Autodesk Inventor part; units mm, degrees
ref_plane "YZ Plane" through (0, 0, 0) normal (1, 0, 0) x (0, 1, 0)
ref_plane "XZ Plane" through (0, 0, 0) normal (0, 1, 0) x (-1, 0, 0)
ref_plane "XY Plane" through (0, 0, 0) normal (0, 0, 1) x (1, 0, 0)
sketch "Sketch1" plane through (0, 0, 0) normal (1, 0, 0) x (0, 1, 0)
  line L0 (32.5, 25) -> (-32.5, 25)
  line L1 (-32.5, 25) -> (-32.5, -25)
  line L2 (-32.5, -25) -> (32.5, -25)
  line L3 (32.5, -25) -> (32.5, 25)
  point P0 (0, 0)
  dimension "d0" = 65
  dimension "d1" = 50
  dimension "d2" = 32.5
  dimension "d3" = 25
extrude "Extrusion1" add sketch "Sketch1" along normal blind 7.5
sketch "Sketch2" plane through (7.5, 0, 0) normal (1, 0, 0) x (0, 0, -1)
  circle A0 centre (-12.5, 20) radius 1.6
  line L0 (25, 32.5) -> (-25, 32.5)
  line L1 (-25, 32.5) -> (-25, -32.5)
  circle A1 centre (12.5, 20) radius 1.6
  line L2 (25, -32.5) -> (25, 32.5)
  point P0 (0, 0)
  dimension "d6" = 3.2
  dimension "d7" = 12.5
  dimension "d8" = 12.5
  dimension "d9" = 3.2
  dimension "d10" = 12.5
  dimension "d11" = 12.5
extrude "Extrusion2" cut sketch "Sketch2" against normal through all
sketch "Sketch3" plane through (7.5, 0, 0) normal (1, 0, 0) x (0, 0, -1)
  circle A0 centre (0, 0) radius 10
  dimension "d14" = 20
extrude "Extrusion3" add sketch "Sketch3" along normal blind 10
sketch "Sketch4" plane through (17.5, 0, 0) normal (1, 0, 0) x (0, 0, -1)
  circle A0 centre (0, 0) radius 5.1
  dimension "d17" = 10.2
extrude "Extrusion4" cut sketch "Sketch4" against normal through all draft -0.75
chamfer "Chamfer1" distance 2 angle 45 6 edges at (7.5, 0, 10) (17.5, 0, 10) (7.5, 0, 25) (7.5, 32.5, 0) (7.5, 0, -25) (7.5, -32.5, 0)
chamfer "Chamfer2" distance 0.5 angle 45 1 edges at (17.5, 0, 5.1)
mirror "Mirror1" about plane through (0, 0, 0) normal (0, 1, 0) of "Extrusion2"
chamfer "Chamfer3" distance 2 angle 45 4 edges at (2.75, 32.5, 25) (2.75, 32.5, -25) (2.75, -32.5, 25) (2.75, -32.5, -25)
sketch "Sketch5" plane through (7.5, 0, 0) normal (1, 0, 0) x (0, 0, -1)
  circle A0 centre (-12.5, 20) radius 1.6
  circle A1 centre (-12.5, 20) radius 3.5
  circle A2 centre (12.5, 20) radius 1.6
  circle A3 centre (12.5, 20) radius 3.5
  circle A4 centre (12.5, -20) radius 1.6
  circle A5 centre (12.5, -20) radius 3.5
  circle A6 centre (-12.5, -20) radius 1.6
  circle A7 centre (-12.5, -20) radius 3.5
  point P0 (0, 0)
  dimension "d29" = 7
  dimension "d30" = 7
  dimension "d31" = 7
  dimension "d32" = 7
extrude "Extrusion5" cut sketch "Sketch5" against normal blind 2.5 contours A0 | A1 | A2 | A3 | A4 | A5 | A6 | A7
properties part number "Front_Cover"
Design review of the part built by this model. Coordinates are the model's own, in mm. A direction names the side the tool comes from. Round coordinates to 2 decimals unless told otherwise and drop trailing zeros. Write each loop counter-clockwise with the first axis right and the second up, starting at its lowest first coordinate (ties: lowest second). Pieces come first, ordered by that corner, then holes. Notation, with made-up numbers: M 64.25,-18 L 117.25,-18 A15 ccw 117.25,10 Z; hole C 27,-36 d11. An arc over 180 degrees is marked long. One line per item, written item: value. Start each with the question number.
1. To check wall thickness, follow probe 1 along Y at (x, z) = (3.7, 12.5); probe 2 along Y at (x, z) = (6.2, -12.5); probe 3 along X at (y, z) = (-5.5, -19). State the ranges of each line that lie inside material, in increasing order. Write a range as from..to.
2. For faces 1 (the face through (6, -32, 0)), 2 (the face through (5, -21, -14)), list the 3-axis set-ups (+Z, -Z, +X, -X, +Y, -Y) from which the entire face can be reached by the end or side of a thin tool; tool diameter is ignored.
3. Take a section at A-A on y = 20. State the section outline as (x, z) points, then the cut area to 3 significant figures.
4. Take a section at C-C on z = 18.5. State the section outline as (x, y) points.
5. Clearance check with flat-ended pins moving along their axes: P1, Ø2, axis at x = 9.5, y = -7.5, coming from the -Z side; P2, Ø8, axis at x = 15, y = -18.5, coming from the +Z side; P3, Ø4, axis at y = 13, z = -16, coming from the +X side; P4, Ø4, axis at y = 20, z = 12.5, coming from the +X side. State where each tip first meets the part, or that it passes through.
6. Draft analysis for pull direction Z (two halves, no side actions). For faces 3 (the face through (17.5, 5.45, 1.89)), 4 (the face through (12.46, 9.76, 2.17)), 5 (the face through (6.27, -16.53, 12.96)), state which applies: pulls with the +Z half, pulls with the -Z half, needs draft (parallel to the pull), parting line crosses it, or undercut.
7. Take a section at B-B on x = 3.5. State the section outline as (y, z) points.
Computed:
1. probe 1: y = -32.5..-21.6, -18.4..18.4, 21.6..32.5
1. probe 2: y = -31.8..-23.5, -16.5..16.5, 23.5..31.8
1. probe 3: x = 0..7.5
2. face 1: +Z, -Z, +X, -Y
2. face 2: +X
3. outline: M 0,-25 L 5.5,-25 L 7.5,-23 L 7.5,-16 L 5,-16 L 5,-14.1 L 0,-14.1 Z; M 0,-10.9 L 5,-10.9 L 5,-9 L 7.5,-9 L 7.5,9 L 5,9 L 5,10.9 L 0,10.9 Z; M 0,14.1 L 5,14.1 L 5,16 L 7.5,16 L 7.5,23 L 5.5,25 L 0,25 Z
3. area: 304 mm²
4. outline: M 0,-32.5 L 5.5,-32.5 L 7.5,-30.5 L 7.5,30.5 L 5.5,32.5 L 0,32.5 Z
5. P1: stops at z = -8.31
5. P2: passes through
5. P3: stops at x = 7.5
5. P4: stops at x = 5
6. face 3: needs draft
6. face 4: parting line crosses it
6. face 5: undercut
7. outline: M -32.5,-23 L -30.5,-25 L 30.5,-25 L 32.5,-23 L 32.5,23 L 30.5,25 L -30.5,25 L -32.5,23 Z; hole C -20,-12.5 d3.2; hole C -20,12.5 d3.2; hole C 0,0 d9.83; hole C 20,-12.5 d3.2; hole C 20,12.5 d3.2
